Design review of the part built by this model. Coordinates are the model's own, in mm. A direction names the side the tool comes from. Give positions to 0.01 mm unless a question says otherwise; leave off trailing zeros. Loops run counter-clockwise (first coordinate to the right, second up) from the corner with the lowest first, then second, coordinate; pieces in that order, holes last.
from build123d import *

# Parameters (mm, degrees)
SKETCH1_W                 = 100
SKETCH1_H                 = 10
BOSS_EXTRUDE1_DEPTH       = 6.35
SKETCH2_W                 = 80
SKETCH2_H                 = 3.175
CUT_EXTRUDE1_DEPTH        = 6.35
F_6_0MM_DOWEL_HOLE1_D     = 6
F_6_0MM_DOWEL_HOLE1_DEPTH = 20
F_6_0MM_DOWEL_HOLE1_TIP   = 1.802581857


with BuildPart() as part:
    # Sketch1 → Boss-Extrude1 (new body)
    with BuildSketch(Plane(origin=(0, 0, 0), x_dir=(1, 0, 0), z_dir=(0, 1, 0))):
        Rectangle(SKETCH1_W, SKETCH1_H)
    extrude(amount=BOSS_EXTRUDE1_DEPTH)

    # Sketch2 → Cut-Extrude1 (cut)
    with BuildSketch(Plane(origin=(0, 6.35, 0), x_dir=(1, 0, 0), z_dir=(0, 1, 0))):
        Rectangle(SKETCH2_W, SKETCH2_H)
    extrude(amount=-CUT_EXTRUDE1_DEPTH, mode=Mode.SUBTRACT)

    # Ø6.0mm Dowel Hole1
    with Locations(Plane(origin=(0, 6.35, 0), x_dir=(1, 0, 0), z_dir=(0, 1, 0))):
        with Locations((-45, 0), (45, 0)):
            Hole(F_6_0MM_DOWEL_HOLE1_D / 2, depth=F_6_0MM_DOWEL_HOLE1_DEPTH)
            with Locations((0, 0, -(F_6_0MM_DOWEL_HOLE1_DEPTH + F_6_0MM_DOWEL_HOLE1_TIP / 2))):  # 118° drill point
                Cone(0, F_6_0MM_DOWEL_HOLE1_D / 2, F_6_0MM_DOWEL_HOLE1_TIP, mode=Mode.SUBTRACT)


solid = part.part
Q1. Wall thickness on line 1 (X direction, y = 2.5, z = -0.25); line 2 (Z direction, x = -15.5, y = 3); line 3 (Z direction, x = 45, y = 4.5): over which ranges is each line inside the solid? List them lowest first.
Results:
line 1: x = -50 to -47.99, -42.01 to -40, 40 to 42.01, 47.99 to 50
line 2: z = -5 to -1.59, 1.59 to 5
line 3: z = -5 to -3, 3 to 5
Q2. Insertion check: pin 1 (4 mm diameter, centred on x = -23.5, z = -1, fed in from -Y). The pin has a flat end and moves straight along its axis. Give the tip position at first contact, or say it passes through.
Results:
pin 1: stops at y = 0
Q3. Take a section at D-D (x = -45). Give the boundary of the cut face in (y, z).
Results:
outline: (0, -5) - (6.35, -5) - (6.35, -3) - (0, -3) - close; (0, 3) - (6.35, 3) - (6.35, 5) - (0, 5) - close
Q4. Take a section at C-C (y = 1). Give the boundary of the cut face in (x, z).
Results:
outline: (-50, -5) - (50, -5) - (50, 5) - (-50, 5) - close; hole circle Ø6 at (-45, 0); hole (-40, -1.59) - (40, -1.59) - (40, 1.59) - (-40, 1.59) - close; hole circle Ø6 at (45, 0)
Q5. Tool access review of faces 1 (the face through (-1, 3, 1.588)), 2 (the face through (-1, 0, -2)): name each direction out of +Z, -Z, +X, -X, +Y, -Y from which nothing blocks a thin tool from reaching the whole face with its end or side.
Results:
face 1: +Y, -Y
face 2: +Z, -Z, +X, -X, -Y
Q6. Take a section at B-B (z = 0). Give the boundary of the cut face in (x, y), plus the area to 3 significant figures.
Results:
outline: (-50, 0) - (-48, 0) - (-48, 6.35) - (-50, 6.35) - close; (-42, 0) - (-40, 0) - (-40, 6.35) - (-42, 6.35) - close; (40, 0) - (42, 0) - (42, 6.35) - (40, 6.35) - close; (48, 0) - (50, 0) - (50, 6.35) - (48, 6.35) - close
area: 50.8 mm2
Q7. Draft analysis for pull direction X (two halves, no side actions). For faces 3 (the face through (-1, 3, -1.588)), 4 (the face through (40, 3, 0)), 5 (the face through (-50, 3, 0)), 6 (the face through (-1, 3, -5)), state which applies: pulls with the +X half, pulls with the -X half, needs draft (parallel to the pull), parting line crosses it, or undercut.
Results:
face 3: undercut
face 4: undercut
face 5: pulls with the -X half
face 6: needs draft
Q8. Take a section at A-A (x = -2). Give the boundary of the cut face in (y, z).
Results:
outline: (0, -5) - (6.35, -5) - (6.35, -1.59) - (0, -1.59) - close; (0, 1.59) - (6.35, 1.59) - (6.35, 5) - (0, 5) - close
